Could you check a few things on this model? Use its own coordinates, in mm. Give positions to 0.01 mm unless a question says otherwise; leave off trailing zeros. Write each loop counter-clockwise with the first axis right and the second up, starting at its lowest first coordinate (ties: lowest second). Pieces come first, ordered by that corner, then holes. Notation, with made-up numbers: M 76,5.25 L 112,5.25 A21 cw 112,18.25 Z; hole C 25,5.25 d11. An arc over 180 degrees is marked long. Use one line per item in the form item = value.
from build123d import *

# Parameters (mm, degrees)
SKETCH1_R           = 4
BOSS_EXTRUDE1_DEPTH = 50
FILLET1_R           = 1
FILLET2_R           = 1


with BuildPart() as part:
    # Sketch1 → Boss-Extrude1 (new body)
    with BuildSketch(Plane(origin=(0, 0, 0), x_dir=(1, 0, 0), z_dir=(0, 1, 0))):
        Circle(SKETCH1_R)
    extrude(amount=BOSS_EXTRUDE1_DEPTH)

    # Fillet1
    fillet1_edges = [part.edges().sort_by_distance(p)[0] for p in [
        (-4, 50, 0),
    ]]
    fillet(fillet1_edges, radius=FILLET1_R)

    # Fillet2
    fillet2_edges = [part.edges().sort_by_distance(p)[0] for p in [
        (-4, 0, 0),
    ]]
    fillet(fillet2_edges, radius=FILLET2_R)


solid = part.part
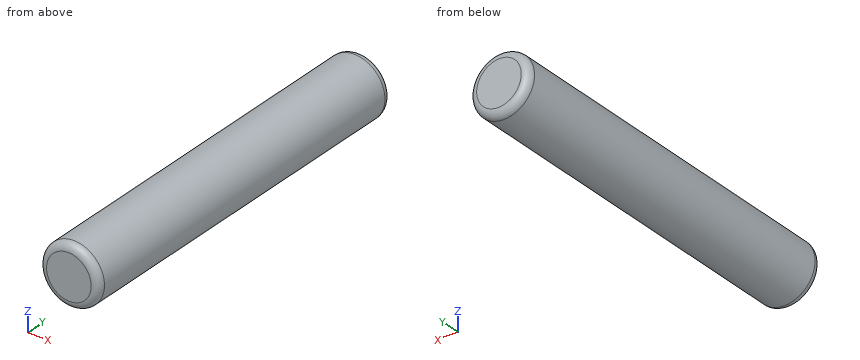
1) I want a section at A-A, the plane y = 44.5. Please give me the cut outline in (x, z).
Checked values:
outline = C 0,0 d8
2) If I drill on L1, parallel to Z at x = -0.25, y = 27; L2, parallel to X at y = 38.5, z = -1.25; L3, parallel to Z at x = -2, y = 10, over which ranges is the centre line in solid material (lowest first)?
Checked values:
L1 = -3.99 to 3.99
L2 = -3.8 to 3.8
L3 = -3.46 to 3.46
3) For pin 1 Ø1.5 at (y, z) = (20, -1) entering from +X; pin 2 Ø1 at (y, z) = (12.5, 1.5) entering from +X, each with a flat end and sliding along its axis, tell me the tip position at first contact or that it passes through.
Checked values:
pin_1 = 3.99
pin_2 = 3.87
